Can you work these out from the model? Positions are in its coordinate system, mm. Face numbers are marked on the shaded views. A direction names the side the tool comes from. Round coordinates to 2 decimals unless told otherwise and drop trailing zeros. Loops run counter-clockwise (first coordinate to the right, second up) from the corner with the lowest first, then second, coordinate; pieces in that order, holes last. Notation, with made-up numbers: (53.25, 40.25) -> (72.25, 40.25) arc R30 cw to (72.25, 72.25) -> close; hole circle Ø4 at (-9.5, 27). An arc over 180 degrees is marked (long way). Write each question's results on one line, items separated by ' | '.
from build123d import *

# Parameters (mm, degrees)
SKETCH1_R           = 6.25
SKETCH1_R_2         = 1.5
BOSS_EXTRUDE1_DEPTH = 3


with BuildPart() as part:
    # Sketch1 → Boss-Extrude1 (new body)
    with BuildSketch(Plane(origin=(0, 0, 0), x_dir=(1, 0, 0), z_dir=(0, 1, 0))):
        Polygon((-42.867412192, 7), (-42.867412192, 10), (-39.867412192, 10), (-39.867412192, 13), (-9.867412192, 13), (-9.867412192, 10), (-6.867412192, 10), (-6.867412192, 7), (-9.867412192, 7), (-9.867412192, 0), (-6.867412192, 0), (-6.867412192, -3), (-9.867412192, -3), (-9.867412192, -6), (-39.867412192, -6), (-39.867412192, -3), (-42.867412192, -3), (-42.867412192, 0), (-39.867412192, 0), (-39.867412192, 7), align=None)
        with Locations((-24.867412192, 3.5)):
            Circle(SKETCH1_R, mode=Mode.SUBTRACT)
        with Locations((-34.867412192, 3.5)):
            Circle(SKETCH1_R_2, mode=Mode.SUBTRACT)
        with Locations((-14.867412192, 3.5)):
            Circle(SKETCH1_R_2, mode=Mode.SUBTRACT)
    extrude(amount=BOSS_EXTRUDE1_DEPTH)


solid = part.part
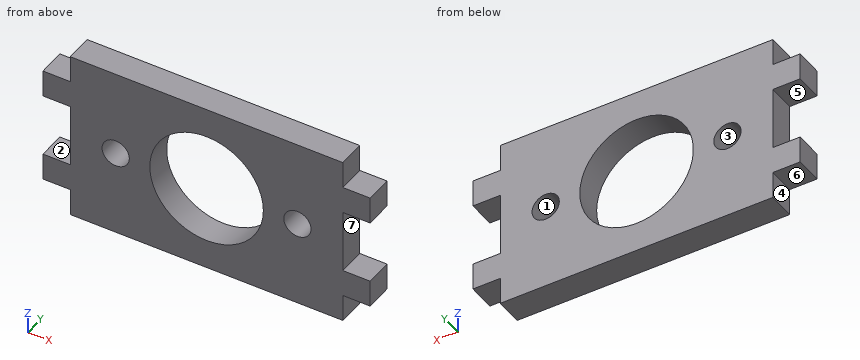
1. If we section it at D-D (z = -7.5): List the corners of the cut face in (x, y) for me.
Final values:
outline: (-42.87, 0) -> (-29.67, 0) -> (-29.67, 3) -> (-42.87, 3) -> close; (-20.07, 0) -> (-6.87, 0) -> (-6.87, 3) -> (-20.07, 3) -> close
2. On a 3-axis mill with a long thin cutter (end or side, diameter ignored), from which of +Z, -Z, +X, -X, +Y, -Y can I reach the whole of each face in a straight line? I mean the marked faces 5, 6 and 7. Say none if no direction works.
Final values:
face 5: -X, +Y, -Y | face 6: -Z, -X, +Y, -Y | face 7: +X, +Y, -Y
3. We'd pull the mould along X, two halves only. Please class the marked faces 1, 2, 3 and 4: pulls with the +X half, pulls with the -X half, needs draft (parallel to the pull), parting line crosses it, or undercut.
Final values:
face 1: undercut | face 2: needs draft | face 3: undercut | face 4: pulls with the -X half
4. Will these pins go through, and if not, where does the flat tip stop? pin 1 (0.9 mm diameter, centred on y = 1, z = -3.5, fed in from -X); pin 2 (2 mm diameter, centred on x = -15.5, z = -4, fed in from +Y); pin 3 (0.9 mm diameter, centred on x = -41, y = 1, fed in from +Z); pin 4 (1.8 mm diameter, centred on x = -14.87, z = -3.5, fed in from +Y).
Final values:
pin 1: x = -39.87 | pin 2: y = 3 | pin 3: z = 3 | pin 4: through
5. If we section it at B-B (x = -15): List the corners of the cut face in (y, z) for me.
Final values:
outline: (0, -13) -> (3, -13) -> (3, -4.99) -> (0, -4.99) -> close; (0, -2.01) -> (3, -2.01) -> (3, 6) -> (0, 6) -> close
6. If we section it at C-C (y = 0.8): List the corners of the cut face in (x, z) for me, then the cut area to 3 significant figures.
Final values:
outline: (-42.87, -10) -> (-39.87, -10) -> (-39.87, -13) -> (-9.87, -13) -> (-9.87, -10) -> (-6.87, -10) -> (-6.87, -7) -> (-9.87, -7) -> (-9.87, 0) -> (-6.87, 0) -> (-6.87, 3) -> (-9.87, 3) -> (-9.87, 6) -> (-39.87, 6) -> (-39.87, 3) -> (-42.87, 3) -> (-42.87, 0) -> (-39.87, 0) -> (-39.87, -7) -> (-42.87, -7) -> close; hole circle Ø3 at (-34.87, -3.5); hole circle Ø12.5 at (-24.87, -3.5); hole circle Ø3 at (-14.87, -3.5) | area: 469 mm2
7. If we section it at A-A (z = -3.5): List the corners of the cut face in (x, y) for me, then the cut area to 3 significant figures.
Final values:
outline: (-39.87, 0) -> (-36.37, 0) -> (-36.37, 3) -> (-39.87, 3) -> close; (-33.37, 0) -> (-31.12, 0) -> (-31.12, 3) -> (-33.37, 3) -> close; (-18.62, 0) -> (-16.37, 0) -> (-16.37, 3) -> (-18.62, 3) -> close; (-13.37, 0) -> (-9.87, 0) -> (-9.87, 3) -> (-13.37, 3) -> close | area: 34.5 mm2
8. Please list where these lines run through material, in increasing order: line 1 (X direction, y = 0.75, z = -3.5); line 2 (Z direction, x = -40, y = 0.9); line 3 (X direction, y = 0.85, z = -4). Write a range as from..to.
Final values:
line 1: -39.87..-36.37, -33.37..-31.12, -18.62..-16.37, -13.37..-9.87 | line 2: -10..-7, 0..3 | line 3: -39.87..-36.28, -33.45..-31.1, -18.64..-16.28, -13.45..-9.87
